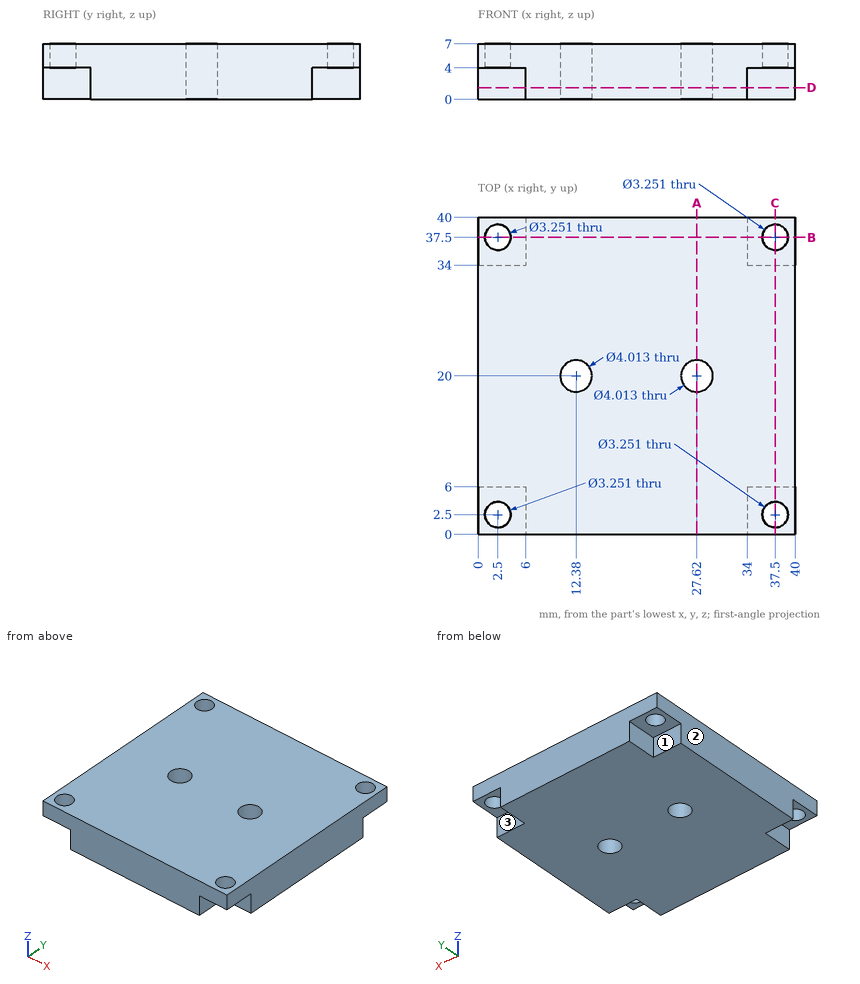
Drawing for the job (mm, zero at the part's lowest x, y, z). A direction names the side the tool comes from. Give positions to 0.01 mm unless a question says otherwise; leave off trailing zeros. Loops run counter-clockwise (first coordinate to the right, second up) from the corner with the lowest first, then second, coordinate; pieces in that order, holes last. Notation, with made-up numbers: M 21,54.5 L 32,54.5 A12 ccw 32,58.5 Z; hole C 82,42 d9. An arc over 180 degrees is marked long. Use one line per item in the form item = value.
Item 1: Slice it at B-B (y = 37.5). List the corners of the cut face in (x, z).
Determined:
outline = M 0,4 L 0.87,4 L 0.87,7 L 0,7 Z; M 4.13,4 L 6,4 L 6,0 L 34,0 L 34,4 L 35.87,4 L 35.87,7 L 4.13,7 Z; M 39.13,4 L 40,4 L 40,7 L 39.13,7 Z
Item 2: Which spindle directions (+Z, -Z, +X, -X, +Y, -Y) get a long thin tool onto all of the face, cutting with end or side? Do the marked faces 1, 2 and 3. Say none if no direction does.
Determined:
face_1 = -Z, -X, +Y
face_2 = +Z, -Z, -X, +Y, -Y
face_3 = -Z, +X, +Y
Item 3: Drill centre lines: probe 1 along X at (y, z) = (2.5, 5.8); probe 2 along X at (y, z) = (2, 5). Where is each one in solid material? Low to high. Write a range as from..to.
Determined:
probe_1 = 0..0.87, 4.13..35.87, 39.13..40
probe_2 = 0..0.95, 4.05..35.95, 39.05..40
Item 4: Flat gauge pins, fed straight in: pin 1 (5 mm diameter, centred on x = 18.5, y = 32, fed in from -Z); pin 2 (3 mm diameter, centred on y = 38, z = 2, fed in from -X); pin 3 (3 mm diameter, centred on x = 12.38, y = 20, fed in from -Z); pin 4 (3.5 mm diameter, centred on x = 37.5, y = 2.5, fed in from -Z). Where does each tip first touch, or does it go through?
Determined:
pin_1 = 0
pin_2 = 6
pin_3 = through
pin_4 = 4
Item 5: Slice it at D-D (z = 1.5). List the corners of the cut face in (x, y), plus the area to 3 significant figures.
Determined:
outline = M 0,6 L 6,6 L 6,0 L 34,0 L 34,6 L 40,6 L 40,34 L 34,34 L 34,40 L 6,40 L 6,34 L 0,34 Z; hole C 12.38,20 d4.01; hole C 27.62,20 d4.01
area = 1,430 mm2
Item 6: Slice it at A-A (x = 27.62). List the corners of the cut face in (y, z).
Determined:
outline = M 0,0 L 17.99,0 L 17.99,7 L 0,7 Z; M 22.01,0 L 40,0 L 40,7 L 22.01,7 Z
